Geometry: final body of the model. Coordinates: model frame, mm. Coordinates: 2 decimals unless noted, no trailing zeros. Order: outer loops, then holes, each group sorted by start corner. A loop starts at its lowest first (then second) coordinate and runs counter-clockwise, first axis right, second up. Notation, with made-up numbers: (-11, -25.5) - (17, -25.5) arc R19 ccw to (17, -3.5) - close; hole circle Ø11 at (74, 85). An arc over 180 degrees is marked (long way). Use a Markdown table: item, result. Add a question column.
```python
from build123d import *

# Parameters (mm, degrees)
SKETCH1_R           = 49.25
BOSS_EXTRUDE1_DEPTH = 2
CUT_EXTRUDE1_DEPTH  = 5


with BuildPart() as part:
    # Sketch1 → Boss-Extrude1 (new body)
    with BuildSketch(Plane(origin=(0, 0, 0), x_dir=(1, 0, 0), z_dir=(0, 1, 0))):
        with BuildLine():
            Line((-134.118891506, 0), (134.118891506, 0))
            ThreePointArc((134.118891506, 0), (137.928249972, 1.76136015), (139.053747558, 5.804484769))
            Line((139.053747558, 5.804484769), (120.84297072, 117.512705691))
            ThreePointArc((120.84297072, 117.512705691), (119.443648574, 120.243754828), (116.712599437, 121.643076974))
            Line((116.712599437, 121.643076974), (84.336583334, 126.921044874))
            ThreePointArc((84.336583334, 126.921044874), (81.605534197, 128.32036702), (80.206212051, 131.051416157))
            Line((80.206212051, 131.051416157), (60.683956749, 250.804484769))
            ThreePointArc((60.683956749, 250.804484769), (58.987740546, 253.809358466), (55.749100697, 255))
            Line((55.749100697, 255), (-55.749100697, 255))
            ThreePointArc((-55.749100697, 255), (-58.987740546, 253.809358466), (-60.683956749, 250.804484769))
            Line((-60.683956749, 250.804484769), (-80.206212051, 131.051416157))
            ThreePointArc((-80.206212051, 131.051416157), (-81.605534197, 128.32036702), (-84.336583334, 126.921044874))
            Line((-84.336583334, 126.921044874), (-116.712599437, 121.643076974))
            ThreePointArc((-116.712599437, 121.643076974), (-119.443648574, 120.243754828), (-120.84297072, 117.512705691))
            Line((-120.84297072, 117.512705691), (-139.053747558, 5.804484769))
            ThreePointArc((-139.053747558, 5.804484769), (-137.928249972, 1.76136015), (-134.118891506, 0))
        make_face()
        with Locations((0, 195)):
            Circle(SKETCH1_R, mode=Mode.SUBTRACT)
        with Locations((-70, 60)):
            Circle(SKETCH1_R, mode=Mode.SUBTRACT)
        with Locations((70, 60)):
            Circle(SKETCH1_R, mode=Mode.SUBTRACT)
    extrude(amount=BOSS_EXTRUDE1_DEPTH)

    # Sketch2 → Cut-Extrude1 (cut)
    with BuildSketch(Plane(origin=(0, 2, 0), x_dir=(1, 0, 0), z_dir=(0, 1, 0))):
        Polygon((-56.088893707, 228.423441568), (-51.568858582, 242.831053531), (-46.559589522, 241.259518139), (-51.079624647, 226.851906177), align=None)
        Polygon((-118.431141418, 12.168946469), (-113.911106293, 26.576558432), (-118.920375353, 28.148093823), (-123.440410478, 13.740481861), align=None)
        Polygon((123.440410478, 13.740481861), (118.920375353, 28.148093823), (113.911106293, 26.576558432), (118.431141418, 12.168946469), align=None)
        Polygon((51.079624647, 226.851906177), (46.559589522, 241.259518139), (51.568858582, 242.831053531), (56.088893707, 228.423441568), align=None)
    extrude(amount=-CUT_EXTRUDE1_DEPTH, mode=Mode.SUBTRACT)


solid = part.part
```
1) Pin query (flat end, axial travel): pin 1 (1 mm diameter, centred on y = 0.5, z = -41, fed in from -X). Return the tip coordinate at first contact, or that it passes through.
2) Section B-B (z = -174). Return loops of the section in (x, y), then the cut area to 3 significant figures.
3) Draft query along Z for faces 1 (the face through (-6.41, 0.99, -243.83)), 2 (the face through (70.58, 0.99, -190.09)), 3 (the face through (-2, 0, -129)), 4 (the face through (-23.024, 0.986, -74.793)). Return one class per face: pulls with the +Z half, pulls with the -Z half, needs draft (parallel to the pull), parting line crosses it, or undercut.
4) Section C-C (z = -104). Return loops of the section in (x, y), then the cut area to 3 significant figures.
5) Ray query, line 1 along X through (y, z) = (1.85, -231.5); line 2 along X through (y, z) = (1.85, -84); line 3 along X through (y, z) = (0.1, -25.5). Return the intervals inside material, ascending.
6) Section A-A (x = 0). Return loops of the section in (y, z), then the cut area to 3 significant figures.
7) Section D-D (y = 1.6). Give the number of separate pieces and of enclosed holes in the cut face, then the cut area to 3 significant figures.
Values follow:
| question | item | result |
|---|---|---|
| 1 | pin 1 | stops at x = -133.4 |
| 2 | outline | (-73.2, 0) - (-44.55, 0) - (-44.55, 2) - (-73.2, 2) - close; (44.55, 0) - (73.2, 0) - (73.2, 2) - (44.55, 2) - close |
| 2 | area | 115 mm² |
| 3 | face 1 | undercut |
| 3 | face 2 | pulls with the -Z half |
| 3 | face 3 | needs draft |
| 3 | face 4 | undercut |
| 4 | outline | (-123.05, 0) - (-92.13, 0) - (-92.13, 2) - (-123.05, 2) - close; (-47.87, 0) - (47.87, 0) - (47.87, 2) - (-47.87, 2) - close; (92.13, 0) - (123.05, 0) - (123.05, 2) - (92.13, 2) - close |
| 4 | area | 315 mm² |
| 5 | line 1 | x = -63.83 to -55.12, -49.62 to -33.07, 33.07 to 49.62, 55.12 to 63.83 |
| 5 | line 2 | x = -126.31 to -113.01, -26.99 to 26.99, 113.01 to 126.31 |
| 5 | line 3 | x = -135.84 to -119.75, -114.25 to -105.15, -34.85 to 34.85, 105.15 to 114.25, 119.75 to 135.84 |
| 6 | outline | (0, -255) - (2, -255) - (2, -244.25) - (0, -244.25) - close; (0, -145.75) - (2, -145.75) - (2, 0) - (0, 0) - close |
| 6 | area | 313 mm² |
| 7 | separate pieces | 1 |
| 7 | enclosed holes | 7 |
| 7 | area | 27,600 mm² |
